The model under review builds one solid part; all positions refer to its coordinate system, in mm. Face numbers are marked on the shaded views. Coordinates: 2 decimals unless noted, no trailing zeros. Loops run counter-clockwise (first coordinate to the right, second up) from the corner with the lowest first, then second, coordinate; pieces in that order, holes last. Notation, with made-up numbers: M -2,38.25 L 34,38.25 A21 cw 34,48.25 Z; hole C -2.5,3.25 d8. An arc over 180 degrees is marked long. Use one line per item in the form item = value.
```python
from build123d import *

# Parameters (mm, degrees)
ESQUISSE1_R        = 3
BOSS_EXTRU_1_DEPTH = 8.5
CONG_1_R           = 1


with BuildPart() as part:
    # Esquisse1 → Boss.-Extru.1 (new body)
    with BuildSketch(Plane.XY):
        with BuildLine():
            Line((0.866025404, 21.490381057), (15.294228634, -3.5))
            ThreePointArc((15.294228634, -3.5), (15.294228634, -4.5), (14.42820323, -5))
            Line((14.42820323, -5), (-14.42820323, -5))
            ThreePointArc((-14.42820323, -5), (-15.294228634, -4.5), (-15.294228634, -3.5))
            Line((-15.294228634, -3.5), (-0.866025404, 21.490381057))
            ThreePointArc((-0.866025404, 21.490381057), (0, 21.990381057), (0.866025404, 21.490381057))
        make_face()
        with Locations((-7.5, 0)):
            Circle(ESQUISSE1_R, mode=Mode.SUBTRACT)
        with Locations((7.5, 0)):
            Circle(ESQUISSE1_R, mode=Mode.SUBTRACT)
        with Locations((0, 12.990381057)):
            Circle(ESQUISSE1_R, mode=Mode.SUBTRACT)
    extrude(amount=BOSS_EXTRU_1_DEPTH)

    # Congé1
    cong_1_edges = [part.edges().sort_by_distance(p)[0] for p in [
        (-15.294228634, -4.5, 8.5),
        (0, -5, 8.5),
        (15.294228634, -4.5, 8.5),
        (8.080127019, 8.995190528, 8.5),
        (0, 21.990381057, 8.5),
        (8.080127019, 8.995190528, 0),
        (15.294228634, -4.5, 0),
        (0, -5, 0),
        (-15.294228634, -4.5, 0),
        (-8.080127019, 8.995190528, 0),
        (0, 21.990381057, 0),
        (-8.080127019, 8.995190528, 8.5),
    ]]
    fillet(cong_1_edges, radius=CONG_1_R)


solid = part.part
```
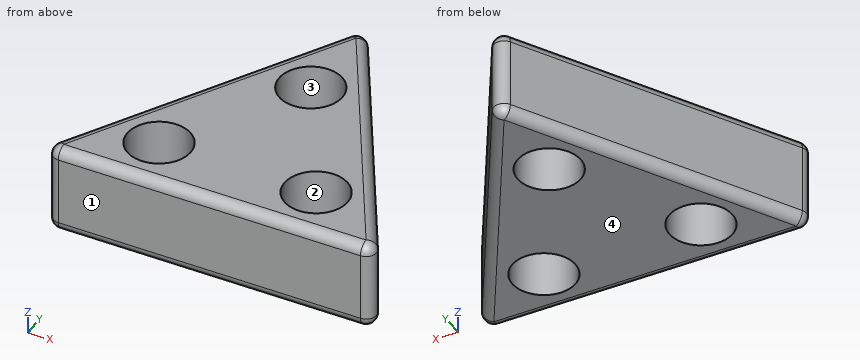
1. The part is to be moulded in two halves that separate along Y. For the marked faces 1, 2, 3 and 4, say which applies: pulls with the +Y half, pulls with the -Y half, needs draft (parallel to the pull), parting line crosses it, or undercut.
Response values:
face_1 = pulls with the -Y half
face_2 = undercut
face_3 = undercut
face_4 = needs draft
2. Add section A-A (z = 2). State the section outline as (x, y) points.
Response values:
outline = M -15.29,-3.5 A1 ccw -14.43,-5 L 14.43,-5 A1 ccw 15.29,-3.5 L 0.87,21.49 A1 ccw -0.87,21.49 Z; hole C -7.5,0 d6; hole C 0,12.99 d6; hole C 7.5,0 d6
3. Add section B-B (y = -2.5). Count the separate pieces of the cut face and the enclosed holes in it, then the cut area to 3 significant figures.
Response values:
separate_pieces = 3
enclosed_holes = 0
area = 193 mm^2
4. Insertion check: P1, Ø3.5, axis at x = 7.5, y = 0, coming from the -Z side; P2, Ø4, axis at x = -5.5, z = 3.5, coming from the +Y side; P3, Ø2, axis at x = 3.5, z = 2, coming from the +Y side. Each pin has a flat end and moves straight along its axis. Give the tip position at first contact, or say it passes through.
Response values:
P1 = through
P2 = 16.93
P3 = 18.66
5. Wall thickness on line 1 along Y through (x, z) = (0, 6); line 2 along X through (y, z) = (-0.5, 5.5); line 3 along X through (y, z) = (-0.75, 7.75): over which ranges is each line inside the solid? List them lowest first. Write a range as from..to.
Response values:
line_1 = -5..9.99, 15.99..21.99
line_2 = -13.56..-10.46, -4.54..4.54, 10.46..13.56
line_3 = -13.67..-10.4, -4.6..4.6, 10.4..13.67
